Here's the drawing with two shaded views (mm, measured from the low corner). I have some questions. A direction names the side the tool comes from. Give positions to 0.01 mm unless a question says otherwise; leave off trailing zeros. Write each loop counter-clockwise with the first axis right and the second up, starting at its lowest first coordinate (ties: lowest second). Pieces come first, ordered by that corner, then holes. Notation, with made-up numbers: M 55.25,35.25 L 65.25,35.25 A34 ccw 65.25,70.25 Z; hole C 1.5,36.5 d5. An arc over 180 degrees is marked long. Answer as a JSON object with one key per item and string values. Group by question number.
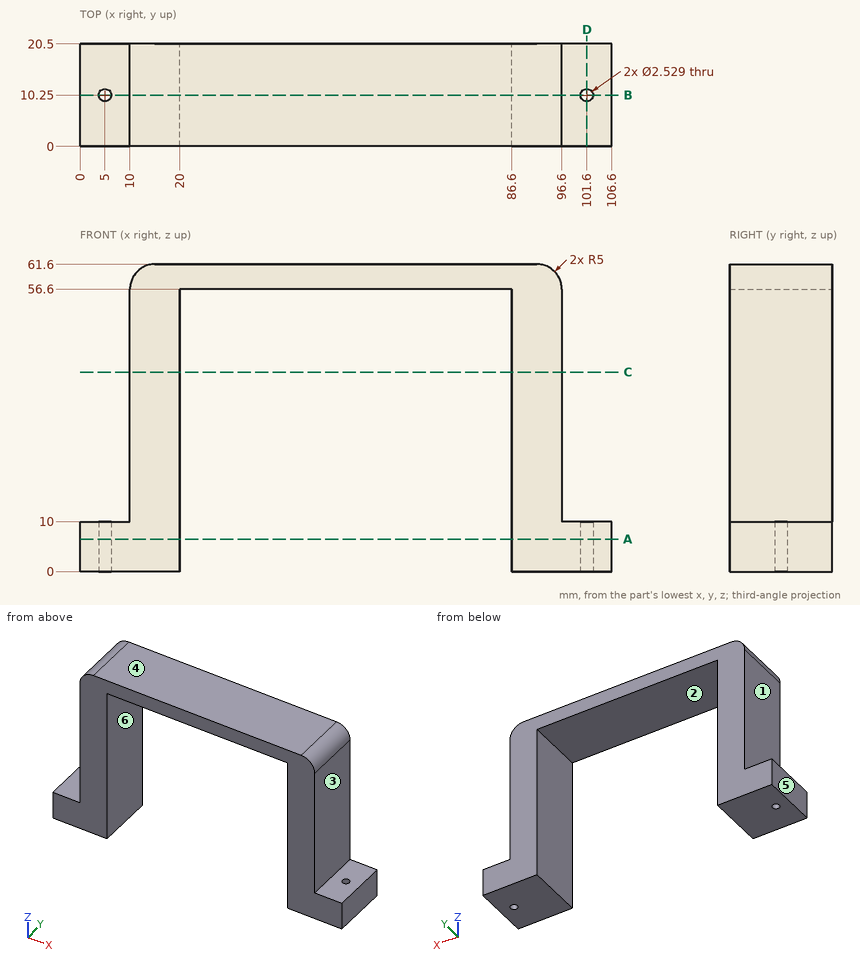
1) I'm going to push flat-ended pins straight in: pin 1 (10 mm diameter, centred on y = 10, z = 45, fed in from -X); pin 2 (8 mm diameter, centred on x = 101.5, y = 14, fed in from +Z); pin 3 (10 mm diameter, centred on y = 4, z = 22, fed in from +X); pin 4 (3.5 mm diameter, centred on x = 5, y = 10.25, fed in from -Z). Where does each tip first touch, or does it pass through?
2) Please list where these lines run through material, in increasing order: line 1 along X through (y, z) = (10.25, 2.25); line 2 along X through (y, z) = (6, 36.5); line 3 along Y through (x, z) = (5, 6). Write a range as from..to.
3) If we section it at A-A, the plane z = 6.5: List the corners of the cut face in (x, y) for me, plus the area to 3 significant figures.
4) For the marked faces 1, 2 and 3, which set-ups out of +Z, -Z, +X, -X, +Y, -Y let a thin tool reach every point of the face, with its end or its side?
5) If we section it at B-B, the plane y = 10.25: List the corners of the cut face in (x, z) for me, plus the area to 3 significant figures.
6) If we section it at D-D, the plane x = 101.6: List the corners of the cut face in (y, z) for me.
7) We'd pull the mould along X, two halves only. Please class the marked faces 4, 5 and 6: released by +X, released by -X, zero draft, split by the parting line, or undercut.
8) If we section it at C-C, the plane z = 40: List the corners of the cut face in (x, y) for me.
Taken from the geometry:
{
 "1": {"pin 1": "x = 10", "pin 2": "z = 10", "pin 3": "x = 96.6", "pin 4": "z = 0"},
 "2": {"line 1": "0..3.74, 6.26..20, 86.6..100.34, 102.86..106.6", "line 2": "10..20, 86.6..96.6", "line 3": "0..8.99, 11.51..20.5"},
 "3": {"outline": "M 0,0 L 20,0 L 20,20.5 L 0,20.5 Z; M 86.6,0 L 106.6,0 L 106.6,20.5 L 86.6,20.5 Z; hole C 5,10.25 d2.53; hole C 101.6,10.25 d2.53", "area": "810 mm²"},
 "4": {"face 1": "+Z, -X, +Y, -Y", "face 2": "-Z, +Y, -Y", "face 3": "+Z, +X, +Y, -Y"},
 "5": {"outline": "M 0,0 L 3.74,0 L 3.74,10 L 0,10 Z; M 6.26,0 L 20,0 L 20,56.6 L 86.6,56.6 L 86.6,0 L 100.34,0 L 100.34,10 L 96.6,10 L 96.6,56.6 A5 ccw 91.6,61.6 L 15,61.6 A5 ccw 10,56.6 L 10,10 L 6.26,10 Z; M 102.86,0 L 106.6,0 L 106.6,10 L 102.86,10 Z", "area": "1,700 mm²"},
 "6": {"outline": "M 0,0 L 8.99,0 L 8.99,10 L 0,10 Z; M 11.51,0 L 20.5,0 L 20.5,10 L 11.51,10 Z"},
 "7": {"face 4": "zero draft", "face 5": "released by -X", "face 6": "undercut"},
 "8": {"outline": "M 10,0 L 20,0 L 20,20.5 L 10,20.5 Z; M 86.6,0 L 96.6,0 L 96.6,20.5 L 86.6,20.5 Z"}
}
